Could you check a few things on this model? Use its own coordinates, in mm. Face numbers are marked on the shaded views. A direction names the side the tool comes from. Round coordinates to 2 decimals unless told otherwise and drop trailing zeros. Order: outer loops, then holes, each group sorted by start corner. A loop starts at its lowest first (then second) coordinate and runs counter-clockwise, first axis right, second up. Notation, with made-up numbers: (53.25, -37) - (110.25, -37) arc R27 cw to (110.25, -7) - close; hole circle Ø3 at (-0.5, 61). An arc over 180 degrees is marked (long way). Use one line per item in the form item = value.
from build123d import *

# Parameters (mm, degrees)
SKETCH_1_W          = 114
SKETCH_1_H          = 56
SKETCH_1_W_2        = 110
SKETCH_1_H_2        = 52
EXTRUDE_1_DEPTH     = 7
SKETCH_2_W          = 114
SKETCH_2_H          = 56
EXTRUDE_1_2_DEPTH   = 1.2
SKETCH_3_R          = 2.5
CUT_EXTRUDE_1_DEPTH = 1.2
FILLET_1_R          = 20
FILLET_2_R          = 21
SKETCH_4_W          = 33.86
SKETCH_4_H          = 14
EXTRUDE_2_DEPTH     = 1.2
SKETCH_5_R          = 2.5
CUT_EXTRUDE_2_DEPTH = 1.2
FILLET_3_R          = 0.1
SKETCH_14_W         = 26
SKETCH_14_H         = 22.2
EXTRUDE_5_DEPTH     = 7
SKETCH_15_W         = 28
SKETCH_15_H         = 18.2
CUT_EXTRUDE_3_DEPTH = 5
SKETCH_18_W         = 2
SKETCH_18_H         = 27
EXTRUDE_6_DEPTH     = 8.2
SKETCH_19_W         = 2
SKETCH_19_H         = 18.2
CUT_EXTRUDE_4_DEPTH = 5
SKETCH_20_R         = 2.5
SKETCH_20_R_2       = 2
CUT_EXTRUDE_5_DEPTH = 5
SKETCH_21_W         = 24
SKETCH_21_H         = 22.2
CUT_EXTRUDE_6_DEPTH = 0.4


with BuildPart() as part:
    # Эскиз1 → Extrude 1 (new body)
    with BuildSketch(Plane.XY):
        Rectangle(SKETCH_1_W, SKETCH_1_H)
        Rectangle(SKETCH_1_W_2, SKETCH_1_H_2, mode=Mode.SUBTRACT)
    extrude(amount=EXTRUDE_1_DEPTH)

    # Эскиз2 → Extrude 1 2 (add)
    with BuildSketch(Plane.XY.offset(7)):
        Rectangle(SKETCH_2_W, SKETCH_2_H)
    extrude(amount=EXTRUDE_1_2_DEPTH)

    # Эскиз3 → Вырез-Вытянуть1 (cut)
    with BuildSketch(Plane.XY.offset(8.2)):
        with Locations((-38.93, 0)):
            Circle(SKETCH_3_R)
        with Locations((-29, 0)):
            Circle(SKETCH_3_R)
        with Locations((-19.07, 0)):
            Circle(SKETCH_3_R)
        with Locations((19.07, 0)):
            Circle(SKETCH_3_R)
        with Locations((29, 0)):
            Circle(SKETCH_3_R)
        with Locations((38.93, 0)):
            Circle(SKETCH_3_R)
    extrude(amount=-CUT_EXTRUDE_1_DEPTH, mode=Mode.SUBTRACT)

    # Скругление1
    fillet_1_edges = [part.edges().sort_by_distance(p)[0] for p in [
        (-55, 26, 3.5),
        (-55, -26, 3.5),
        (55, -26, 3.5),
        (55, 26, 3.5),
    ]]
    fillet(fillet_1_edges, radius=FILLET_1_R)

    # Скругление2
    fillet_2_edges = [part.edges().sort_by_distance(p)[0] for p in [
        (-57, 28, 4.1),
        (57, 28, 4.1),
        (57, -28, 4.1),
        (-57, -28, 4.1),
    ]]
    fillet(fillet_2_edges, radius=FILLET_2_R)

    # Эскиз4 → Бобышка-Вытянуть2 (add)
    with BuildSketch(Plane(origin=(0, 0, 7), x_dir=(-1, 0, 0), z_dir=(0, 0, -1))):
        with Locations((29, 0)):
            Rectangle(SKETCH_4_W, SKETCH_4_H)
        with Locations((-29, 0)):
            Rectangle(SKETCH_4_W, SKETCH_4_H)
    extrude(amount=EXTRUDE_2_DEPTH)

    # Эскиз5 → Вырез-Вытянуть2 (cut)
    with BuildSketch(Plane.XY.offset(7)):
        with Locations((-29, 0)):
            Circle(SKETCH_5_R)
        with Locations((-38.93, 0)):
            Circle(SKETCH_5_R)
        with Locations((-19.07, 0)):
            Circle(SKETCH_5_R)
        with Locations((19.07, 0)):
            Circle(SKETCH_5_R)
        with Locations((29, 0)):
            Circle(SKETCH_5_R)
        with Locations((38.93, 0)):
            Circle(SKETCH_5_R)
    extrude(amount=-CUT_EXTRUDE_2_DEPTH, mode=Mode.SUBTRACT)

    # Скругление3
    fillet_3_edges = [part.edges().sort_by_distance(p)[0] for p in [
        (36.43, 0, 5.8),
        (16.57, 0, 5.8),
        (-21.57, 0, 5.8),
        (-41.43, 0, 5.8),
    ]]
    fillet(fillet_3_edges, radius=FILLET_3_R)

    # Эскиз14 → Бобышка-Вытянуть5 (add)
    with BuildSketch(Plane(origin=(0, 0, 7), x_dir=(-1, 0, 0), z_dir=(0, 0, -1))):
        with Locations((68, 1.5)):
            Rectangle(SKETCH_14_W, SKETCH_14_H)
    extrude(amount=EXTRUDE_5_DEPTH)

    # Эскиз15 → Вырез-Вытянуть3 (cut)
    with BuildSketch(Plane(origin=(0, 0, 0), x_dir=(-1, 0, 0), z_dir=(0, 0, -1))):
        with Locations((67, 1.5)):
            Rectangle(SKETCH_15_W, SKETCH_15_H)
    extrude(amount=-CUT_EXTRUDE_3_DEPTH, mode=Mode.SUBTRACT)

    # Эскиз18 → Бобышка-Вытянуть6 (add)
    with BuildSketch(Plane.XY.offset(8.2)):
        with Locations((-56, 1.5)):
            Rectangle(SKETCH_18_W, SKETCH_18_H)
    extrude(amount=-EXTRUDE_6_DEPTH)

    # Эскиз19 → Вырез-Вытянуть4 (cut)
    with BuildSketch(Plane(origin=(0, 0, 0), x_dir=(-1, 0, 0), z_dir=(0, 0, -1))):
        with Locations((56, 1.5)):
            Rectangle(SKETCH_19_W, SKETCH_19_H)
    extrude(amount=-CUT_EXTRUDE_4_DEPTH, mode=Mode.SUBTRACT)

    # Эскиз20 → Вырез-Вытянуть5 (cut)
    with BuildSketch(Plane(origin=(0, 0, 5), x_dir=(-1, 0, 0), z_dir=(0, 0, -1))):
        with Locations((68.5, 0)):
            Circle(SKETCH_20_R)
        with Locations((68.5, 6)):
            Circle(SKETCH_20_R_2)
    extrude(amount=-CUT_EXTRUDE_5_DEPTH, mode=Mode.SUBTRACT)

    # Эскиз21 → Вырез-Вытянуть6 (cut)
    with BuildSketch(Plane.XY.offset(7)):
        with Locations((-69, 1.5)):
            Rectangle(SKETCH_21_W, SKETCH_21_H)
    extrude(amount=-CUT_EXTRUDE_6_DEPTH, mode=Mode.SUBTRACT)


solid = part.part
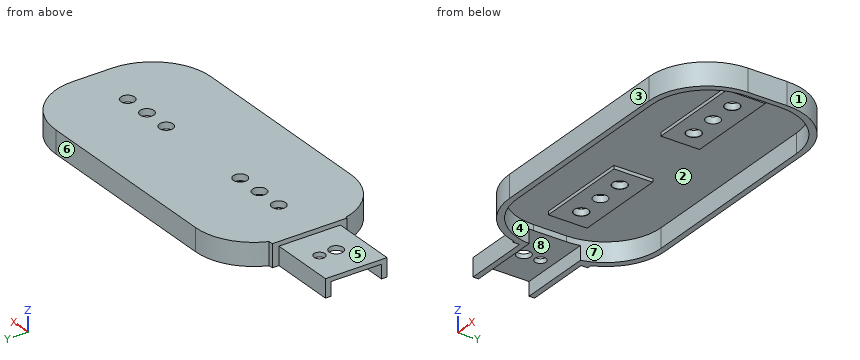
Item 1: For the marked faces 5, 6, 7 and 8, which set-ups out of +Z, -Z, +X, -X, +Y, -Y let a thin tool reach every point of the face, with its end or its side?
Found:
face_5 = +Z, -X, +Y, -Y
face_6 = +Z, -Z, +X, -X, +Y
face_7 = -Z
face_8 = -Z, -X
Item 2: Will these pins go through, and if not, where does the flat tip stop? P1, Ø4, axis at x = -72.5, z = 1.5, coming from the -Y side; P2, Ø11, axis at x = -34.5, y = -2.5, coming from the -Z side; P3, Ø3, axis at y = -21.5, z = 2, coming from the +X side.
Found:
P1 = -9.6
P2 = 5.8
P3 = 52.49
Item 3: Imagine slicing it at A-A on x = -68.5. Please give me the cut outline in (y, z).
Found:
outline = (-9.6, 0) - (-7.6, 0) - (-7.6, 5) - (-2.5, 5) - (-2.5, 6.6) - (-9.6, 6.6) - close; (2.5, 5) - (4, 5) - (4, 6.6) - (2.5, 6.6) - close; (8, 5) - (10.6, 5) - (10.6, 0) - (12.6, 0) - (12.6, 6.6) - (8, 6.6) - close
Item 4: If we mould it in two halves opening along X, with no side actions, what happens to the marked faces 1, 2, 3 and 4? For each: released by +X, released by -X, zero draft, split by the parting line, or undercut.
Found:
face_1 = released by +X
face_2 = undercut
face_3 = zero draft
face_4 = undercut
Item 5: I need wall thicknesses on L1, parallel to Y at x = -68.5, z = 5.6; L2, parallel to Y at x = -10, z = 5.5; L3, parallel to Y at x = -19.07, z = 7.6. Which ranges of each line are inside material? Lowest first, please.
Found:
L1 = -9.6 to -2.5, 2.5 to 4, 8 to 12.6
L2 = -28 to -26, 26 to 28
L3 = -28 to -2.5, 2.5 to 28
Item 6: Imagine slicing it at C-C on y = -4.5. Please give me the cut outline in (x, z).
Found:
outline = (-81, 5) - (-55, 5) - (-55, 7) - (-45.93, 7) - (-45.93, 5.8) - (-12.07, 5.8) - (-12.07, 7) - (12.07, 7) - (12.07, 5.8) - (45.93, 5.8) - (45.93, 7) - (55, 7) - (55, 0) - (57, 0) - (57, 8.2) - (-57, 8.2) - (-57, 6.6) - (-81, 6.6) - close
Item 7: Imagine slicing it at B-B on x = 29. Please give me the cut outline in (y, z), plus the area to 3 significant figures.
Found:
outline = (-28, 0) - (-26, 0) - (-26, 7) - (-7, 7) - (-7, 5.8) - (-2.5, 5.8) - (-2.5, 8.2) - (-28, 8.2) - close; (2.5, 5.8) - (7, 5.8) - (7, 7) - (26, 7) - (26, 0) - (28, 0) - (28, 8.2) - (2.5, 8.2) - close
area = 100 mm2
Item 8: Imagine slicing it at D-D on x = -25. Please give me the cut outline in (y, z), plus the area to 3 significant figures.
Found:
outline = (-28, 0) - (-26, 0) - (-26, 7) - (-7, 7) - (-7, 5.8) - (7, 5.8) - (7, 7) - (26, 7) - (26, 0) - (28, 0) - (28, 8.2) - (-28, 8.2) - close
area = 112 mm2
